Geometry: final body of the model. Coordinates: model frame, mm. Face numbers are marked on the shaded views. A direction names the side the tool comes from. Coordinates: 2 decimals unless noted, no trailing zeros. Order: outer loops, then holes, each group sorted by start corner. A loop starts at its lowest first (then second) coordinate and runs counter-clockwise, first axis right, second up. Notation, with made-up numbers: (74, -9) - (120, -9) arc R36 ccw to (120, 30) - close; hole circle Ø10 at (-14, 72). An arc over 180 degrees is marked (long way). Use one line per item in the form item = value. Start each with the question number.
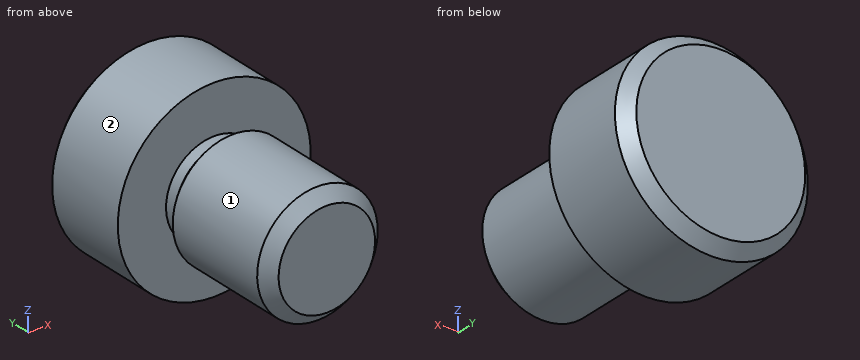
```python
from build123d import *

# Parameters (mm, degrees)
CHAMFER_1_SIZE = 1


with BuildPart() as part:
    # 草图1 → 旋转1 (revolve)
    with BuildSketch(Plane.XY, mode=Mode.PRIVATE) as revolve_1_sk:
        Polygon((0, 0), (8, 0), (8, -8), (4, -8), (4, -9), (5, -9), (5, -20), (0, -20), align=None)
    revolve(revolve_1_sk.sketch.rotate(Axis((0, -20, 0), (0, 1, 0)), 90), axis=Axis((0, -20, 0), (0, 1, 0)))

    # 倒角1
    chamfer_1_edges = [part.edges().sort_by_distance(p)[0] for p in [
        (0, -20, 5),
        (0, -9, 5),
        (0, 0, 8),
    ]]
    chamfer(chamfer_1_edges, length=CHAMFER_1_SIZE - 0.0001)  # a hair under: the kernel refuses the full size


solid = part.part
```
(1) Cut plane D-D on y = -11. Return the cut outline in (x, z), plus the area to 3 significant figures.
(2) Contact query for flat-ended pins moving along their axis: pin 1 Ø3 at (y, z) = (-5, 5) entering from -X; pin 2 Ø2 at (y, z) = (-15, 4) entering from -X; pin 3 Ø4 at (y, z) = (-4.5, 3) entering from -X. Output: stop coordinate, or through.
(3) Cut plane C-C on y = -5.5. Return the cut outline in (x, z), plus the area to 3 significant figures.
(4) Material intervals for L1, parallel to Y at x = -3.25, z = 4; L2, parallel to Z at x = 0.25, y = -11; L3, parallel to Y at x = -4.75, z = 1, sorted ascending. Write a range as from..to.
(5) Set-up query: the marked faces 1 and 2. Return all of +Z, -Z, +X, -X, +Y, -Y with unobstructed straight access to the full face (end or side cutting, diameter ignored); none if empty.
Check sheet entries:
q1.outline = circle Ø10 at (0, 0)
q1.area = 78.5 mm^2
q2.pin_1 = -7.19
q2.pin_2 = -4
q2.pin_3 = -7.94
q3.outline = circle Ø16 at (0, 0)
q3.area = 201 mm^2
q4.L1 = -8..0
q4.L2 = -4.99..4.99
q4.L3 = -19.15..-9.85, -8..0
q5.face_1 = -Y
q5.face_2 = +Y, -Y
